Here's how the part is built. I have some questions about the finished solid (model axes, mm). Face numbers are marked on the shaded views. A direction names the side the tool comes from. Round coordinates to 2 decimals unless told otherwise and drop trailing zeros. Order: outer loops, then holes, each group sorted by start corner. A loop starts at its lowest first (then second) coordinate and runs counter-clockwise, first axis right, second up.
Autodesk Inventor part; units mm, degrees
ref_plane "YZ Plane" through (0, 0, 0) normal (1, 0, 0) x (0, 1, 0)
ref_plane "XZ Plane" through (0, 0, 0) normal (0, 1, 0) x (-1, 0, 0)
ref_plane "XY Plane" through (0, 0, 0) normal (0, 0, 1) x (1, 0, 0)
sketch "Boceto1" plane through (0, 0, 0) normal (0, 0, 1) x (1, 0, 0)
  line L0 (42.8032, 3.438) -> (42.2388, 3.4264) construction
  line L1 (32.2478, 2.8886) -> (18.1678, 2.1307)
  line L2 (8.5818, 18.9887) -> (9.1664, 18.0334)
  line L3 (9.1664, 18.0334) -> (52.8836, 15.3138)
  arc A0 (54.0881, 17.2258) -> (54.0687, 17.2439) centre (52.0315, 15.0417) ccw
  line L4 (54.0687, 17.2439) -> (8.6649, 20.0685)
  line L5 (8.6649, 20.0685) -> (8.3833, 19.5786)
  line L6 (8.3833, 19.5786) -> (8.5818, 18.9887)
  line L7 (17.0583, 0.068) -> (31.7076, 0.8566)
  line L8 (17.0583, 0.068) -> (18.1678, 2.1307)
  arc A1 (53.8325, 16.6216) -> (52.8836, 15.3138) centre (54.4554, 15.1715) ccw
  line L9 (53.8325, 16.6216) -> (54.0881, 17.2258)
  line L10 (32.2478, 2.8886) -> (18.1678, 2.1307)
  line L11 (18.1678, 2.1307) -> (33.7743, 2.9708)
  line L12 (33.7743, 2.9708) -> (34.9191, 2.9708)
  line L13 (34.9191, 2.9708) -> (34.4156, 1.0024)
  line L14 (34.4156, 1.0024) -> (31.7076, 0.8566)
  point P0 (0, 0)
  point P1 (23.6867, 2.4277)
  point P2 (23.6867, 2.4277)
  point P3 (34.3467, 2.9708)
  dimension "d40" = 2
  dimension "d41" = 2
extrude "Extrusión1" add sketch "Boceto1" against normal blind 6.5
sketch "Boceto2" plane through (0, 0, 0) normal (0, 0, 1) x (1, 0, 0)
  line L0 (8.9388, 9.1447) -> (47.9388, 9.1447) construction
  line L1 (51.4388, 12.1447) -> (51.4388, 15.3947) construction
  line L2 (9.1664, 16.6413) -> (8.4891, 17.498)
  line L3 (8.4891, 17.498) -> (9.1664, 18.0334)
  line L4 (9.1664, 18.0334) -> (52.8836, 15.3138)
  line L5 (33.7743, 2.9708) -> (18.1678, 2.1307)
  arc A0 (18.1678, 2.1307) -> (9.1664, 16.6413) centre (4.1736, 3.4968) ccw
  line L6 (18.1678, 2.1307) -> (33.7743, 2.9708)
  line L7 (33.7743, 2.9708) -> (37.722, 2.9708)
  arc A1 (51.2828, 14.4758) -> (37.722, 2.9708) centre (50.5158, 1.6354) ccw
  line L8 (52.8836, 15.3138) -> (53.5092, 15.187)
  line L9 (53.5092, 15.187) -> (53.4837, 14.7773)
  line L10 (53.4837, 14.7773) -> (51.2828, 14.4758)
  point P0 (0, 0)
  point P1 (1.4388, 9.1447)
  point P2 (23.6867, 2.4277)
  point P3 (51.9388, 13.5511)
  point P4 (32.2478, 2.8886)
  point P5 (40.9403, 9.1447)
  point P6 (32.2478, 2.8886)
  dimension "d27" = 3.5
  dimension "d31" = 3.25
extrude "Extrusión2" add sketch "Boceto2" against normal blind 1
properties part number "Pieza1_Carcasa_3DPrint"
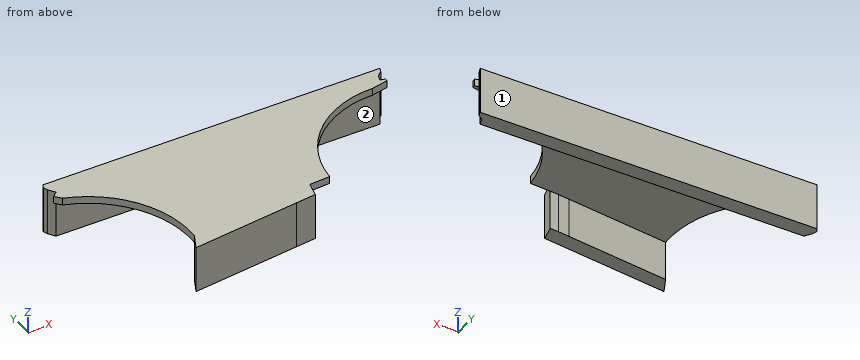
1. I'm going to push flat-ended pins straight in: P1, Ø4, axis at x = 16.5, y = 15.5, coming from the +Z side; P2, Ø0.8, axis at x = 35.5, z = -0.5, coming from the -Y side. Where does each tip first touch, or does it pass through?
Evaluation:
P1: stops at z = 0
P2: stops at y = 2.97
2. I need wall thicknesses on probe 1 along Y at (x, z) = (23, -6); probe 2 along Z at (x, y) = (19, 5.75); probe 3 along Y at (x, z) = (24, -4.75). Which ranges of each line are inside material? Lowest first, please.
Evaluation:
probe 1: y = 0.39 to 2.39, 17.17 to 19.18
probe 2: z = -1 to 0
probe 3: y = 0.44 to 2.44, 17.11 to 19.11
3. If we section it at B-B, the plane x = 33: Write out the boundary of the cut face in (y, z).
Evaluation:
outline: (0.93, -6.5) - (2.93, -6.5) - (2.93, -1) - (16.55, -1) - (16.55, -6.5) - (18.55, -6.5) - (18.55, 0) - (0.93, 0) - close
4. If we section it at D-D, the plane x = 22: Write out the boundary of the cut face in (y, z), and give its area (3 significant figures).
Evaluation:
outline: (0.33, -6.5) - (2.34, -6.5) - (2.34, -1) - (17.24, -1) - (17.24, -6.5) - (19.24, -6.5) - (19.24, 0) - (0.33, 0) - close
area: 40.9 mm2
5. If we section it at C-C, the plane y = 8.5: Write out the boundary of the cut face in (x, z).
Evaluation:
outline: (17.31, -1) - (39.64, -1) - (39.64, 0) - (17.31, 0) - close
6. On a 3-axis mill with a long thin cutter (end or side, diameter ignored), from which of +Z, -Z, +X, -X, +Y, -Y can I reach the whole of each face in a straight line? I mean the marked faces 1 and 2. Say none if no direction works.
Evaluation:
face 1: +Z, -Z, +X, +Y
face 2: -Z, -X
